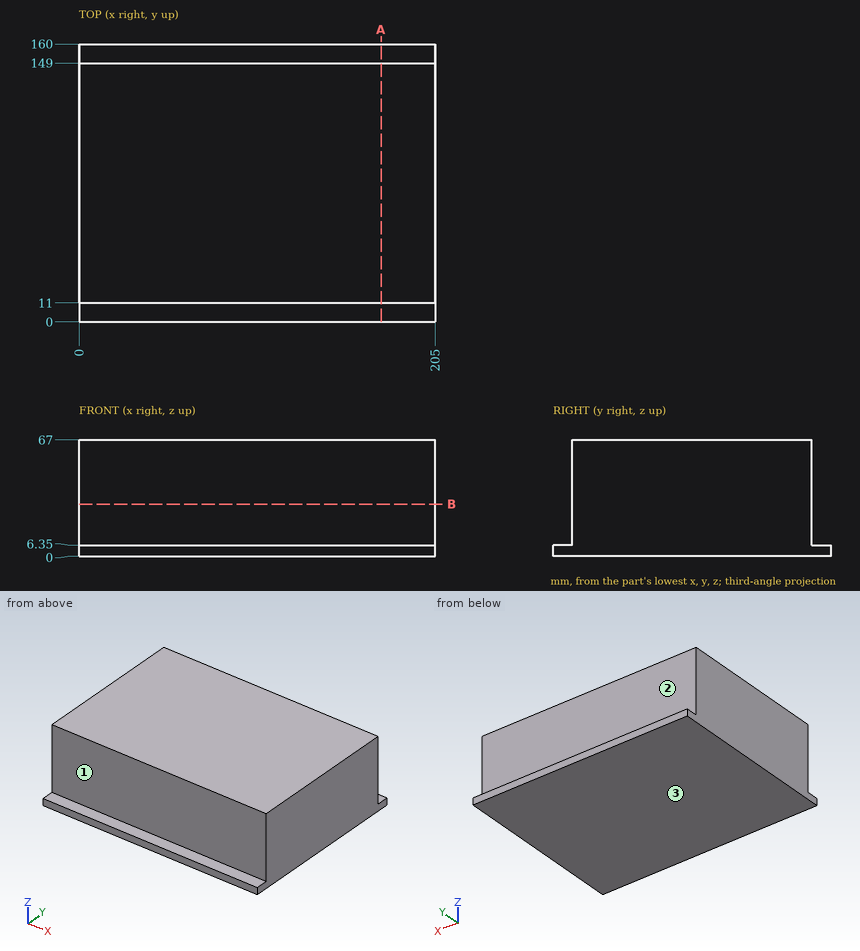
Job drawing, mm, ordinate dimensions from the low corner. One solid piece. A direction names the side the tool comes from. Round coordinates to 2 decimals unless told otherwise and drop trailing zeros. Write each loop counter-clockwise with the first axis right and the second up, starting at its lowest first coordinate (ties: lowest second). Pieces come first, ordered by that corner, then holes. Notation, with made-up numbers: M 69,-26.75 L 84,-26.75 A31 cw 84,6.25 Z; hole C 51.5,79.5 d7. An arc over 180 degrees is marked long. Return JSON: item names as keys, results as strings. Group by question number.
(1) Which spindle directions (+Z, -Z, +X, -X, +Y, -Y) get a long thin tool onto all of the face, cutting with end or side? Do the marked faces 1, 2 and 3. Say none if no direction does.
(2) Saw through at A-A on x = 174. Write the cut outline in (y, z).
(3) Pin check, flat tips, straight feed: pin 1 Ø3.5 at (x, y) = (53, 156.5) entering from +Z; pin 2 Ø6 at (x, z) = (139, 11) entering from -Y; pin 3 Ø4 at (x, z) = (57, 19) entering from +Y; pin 4 Ø5 at (y, z) = (84.5, 41) entering from -X. Stop position of each tip, or through.
(4) Saw through at B-B on z = 30. Write the cut outline in (x, y), then the cut area to 3 significant figures.
(5) Drill centre lines: probe 1 along Z at (x, y) = (178.5, 152); probe 2 along Y at (x, z) = (47, 63). Where is each one in solid material? Low to high.
Returned:
{
 "1": {"face 1": "+Z, +X, -X, -Y", "face 2": "+Z, +X, -X, +Y", "face 3": "-Z, +X, -X, +Y, -Y"},
 "2": {"outline": "M 0,0 L 160,0 L 160,6.35 L 149,6.35 L 149,67 L 11,67 L 11,6.35 L 0,6.35 Z"},
 "3": {"pin 1": "z = 6.35", "pin 2": "y = 11", "pin 3": "y = 149", "pin 4": "x = 0"},
 "4": {"outline": "M 0,11 L 205,11 L 205,149 L 0,149 Z", "area": "28,300 mm²"},
 "5": {"probe 1": "0 to 6.35", "probe 2": "11 to 149"}
}
